The listing builds one solid part. Answer for the finished solid, in the listing's coordinates (mm). A direction names the side the tool comes from. Coordinates: 2 decimals unless noted, no trailing zeros. Loops run counter-clockwise (first coordinate to the right, second up) from the corner with the lowest first, then second, coordinate; pieces in that order, holes last. Notation, with made-up numbers: M 29,-35 L 60,-35 A18 cw 60,-5 Z; hole C 54,42.5 d4. An arc over 180 degrees is marked long. Return JSON: item names as keys, results as strings. Group by question number.
1. The mould has two halves that part along X. Classify faces 6 (the face through (0, 28, 1)), 7 (the face through (-0.65, -13.07, 9.97)), 8 (the face through (28, 0, 1)), 9 (the face through (13.65, 15.18, 10.23)): pulls with the +X half, pulls with the -X half, needs draft (parallel to the pull), parting line crosses it, or undercut.
2. Section D-D (x = -16) is taken. Write down the section's boundary in (y, z).
3. Given P1, Ø1.8, axis at y = 19.5, z = 10.5, coming from the +X side; P2, Ø10, axis at x = 4, y = 3.5, coming from the -Z side; P3, Ø3, axis at y = 3, z = 5, coming from the -X side; P4, Ø4, axis at x = -21.5, z = 6.5, coming from the +Y side, each flat-ended and moving along its own axis, determine where each tip first touches the part or whether it passes through.
4. Straight lines are drawn through the part: L1, parallel to X at y = -23, z = 2.3; L2, parallel to Z at x = 1.5, y = -7. For each, find the intervals that lie inside material, in ascending order. Write a range as from..to.
5. Section C-C (y = -15.25) is taken. Write down the section's boundary in (x, z), then the cut area to 3 significant figures.
6. Which of the six approach directions +Z, -Z, +X, -X, +Y, -Y give full straight-line access (tool end or side, diameter ignored) to faces 1 (the face through (0, 0, 3)), 2 (the face through (17, 11, 10)), 3 (the face through (13, 0, 10)), 4 (the face through (21, -8, 10)), 5 (the face through (0, -21, 10))?
7. Section A-A (x = 23) is taken. Write down the section's boundary in (y, z).
8. Section B-B (z = 10.75) is taken. Count the separate pieces of the cut face and the enclosed holes in it, then the cut area to 3 significant figures.
Autodesk Fusion 360 part; units mm, degrees
sketch "Sketch1" plane through (0, 0, 0) normal (0, 0, 1) x (1, 0, 0) in component "FC_TRAY_V1"
  line L0 (-28, -28) -> (28, -28)
  line L1 (28, -28) -> (28, 28)
  line L2 (28, 28) -> (-28, 28)
  line L3 (-28, 28) -> (-28, -28)
extrude "Extrude1" add sketch "Sketch1" along normal blind 3 makes body 1 in component "FC_TRAY_V1"
sketch "Sketch2" plane through (0, 0, 0) normal (0, 0, 1) x (1, 0, 0) in component "FC_TRAY_V1"
  circle A0 centre (16, 0) radius 4
  circle A1 centre (-16, 0) radius 4
  circle A2 centre (0, 16) radius 4
  circle A3 centre (0, -16) radius 4
extrude "Extrude2" add sketch "Sketch2" along normal blind 6.5 from surface at 2.5 separate body makes body 2 at (19.9801, -0.3983, 6.8333) makes body 3 at (3.9801, 15.6017, 6.8333) makes body 4 at (-12.0199, -0.3983, 6.8333) makes body 5 at (3.9801, -16.3983, 6.8333) in component "FC_TRAY_V1"
sketch "Sketch3" plane through (0, 0, 0) normal (0, 0, 1) x (1, 0, 0) in component "FC_TRAY_V1"
  line L0 (-21, -21) -> (21, -21)
  line L1 (21, -21) -> (21, 21)
  line L2 (21, 21) -> (-21, 21)
  line L3 (-21, 21) -> (-21, -21)
extrude "Extrude3" add sketch "Sketch3" along normal blind 3.5 from surface at 8.5 separate body makes body 6 in component "FC_TRAY_V1"
combine "Combine1" operation add target body 1 tool bodies 2 3 4 5 6 in component "FC_TRAY_V1"
sketch "Sketch4" plane through (0, 0, 0) normal (0, 0, 1) x (1, 0, 0) in component "FC_TRAY_V1"
  circle A0 centre (23, 23) radius 1.7
  circle A1 centre (-23, 23) radius 1.7
  circle A2 centre (23, -23) radius 1.7
  circle A3 centre (-23, -23) radius 1.7
extrude "Extrude4" cut sketch "Sketch4" along normal blind 5 from surface at -1 bodies 1 in component "FC_TRAY_V1"
sketch "Sketch5" plane through (0, 0, 0) normal (0, 0, 1) x (1, 0, 0) in component "FC_TRAY_V1"
  circle A0 centre (15.25, 15.25) radius 1.6
  circle A1 centre (-15.25, 15.25) radius 1.6
  circle A2 centre (15.25, -15.25) radius 1.6
  circle A3 centre (-15.25, -15.25) radius 1.6
extrude "Extrude5" cut sketch "Sketch5" along normal blind 5 from surface at 8 bodies 1 in component "FC_TRAY_V1"
sketch "Sketch6" plane through (0, 0, 0) normal (0, 0, 1) x (1, 0, 0) in component "FC_TRAY_V1"
  circle A0 centre (16, 0) radius 3
  circle A1 centre (-16, 0) radius 3
  circle A2 centre (0, 16) radius 3
  circle A3 centre (0, -16) radius 3
extrude "Extrude6" cut sketch "Sketch6" along normal blind 4 from surface at 8 bodies 1 in component "FC_TRAY_V1"
sketch "Sketch7" plane through (0, 0, 0) normal (0, 0, 1) x (1, 0, 0) in component "FC_TRAY_V1"
  line L0 (17, 6) -> (21, 6)
  line L1 (21, 6) -> (21, 16)
  line L2 (21, 16) -> (17, 16)
  line L3 (17, 16) -> (17, 6)
extrude "Extrude7" cut sketch "Sketch7" along normal blind 5 from surface at 8 bodies 1 in component "FC_TRAY_V1"
component "FC_TRAY_V1" placed x (1, 0, 0) y (0, 1, 0) z (0, 0, 1) at (0, 0, 0)
Worked out:
{
 "1": {"face 6": "needs draft", "face 7": "undercut", "face 8": "pulls with the +X half", "face 9": "undercut"},
 "2": {"outline": "M -28,0 L 28,0 L 28,3 L 4,3 L 4,8.5 L 13.84,8.5 L 13.84,12 L 3,12 L 3,8 L -3,8 L -3,12 L -13.84,12 L -13.84,8.5 L -4,8.5 L -4,3 L -28,3 Z; M -21,8.5 L -16.66,8.5 L -16.66,12 L -21,12 Z; M 16.66,8.5 L 21,8.5 L 21,12 L 16.66,12 Z"},
 "3": {"P1": "x = 21", "P2": "z = 0", "P3": "x = -19.71", "P4": "y = 1.94"},
 "4": {"L1": "-28..-24.7, -21.3..21.3, 24.7..28", "L2": "0..3, 8.5..12"},
 "5": {"outline": "M -28,0 L 28,0 L 28,3 L 3.93,3 L 3.93,8.5 L 13.65,8.5 L 13.65,12 L 2.9,12 L 2.9,8 L -2.9,8 L -2.9,12 L -13.65,12 L -13.65,8.5 L -3.93,8.5 L -3.93,3 L -28,3 Z; M -21,8.5 L -16.85,8.5 L -16.85,12 L -21,12 Z; M 16.85,8.5 L 21,8.5 L 21,12 L 16.85,12 Z", "area": "313 mm^2"},
 "6": {"face 1": "none", "face 2": "+Z, +X", "face 3": "+Z", "face 4": "+Z, +X, +Y, -Y", "face 5": "+Z, +X, -X, -Y"},
 "7": {"outline": "M -28,0 L -24.7,0 L -24.7,3 L -28,3 Z; M -21.3,0 L 21.3,0 L 21.3,3 L -21.3,3 Z; M 24.7,0 L 28,0 L 28,3 L 24.7,3 Z"},
 "8": {"separate pieces": "1", "enclosed holes": "8", "area": "1,580 mm^2"}
}
